Autodesk Inventor part; units mm, degrees
ref_plane "Plano de trabajo1" through (120, 0, 0) normal (1, 0, 0) x (0, 1, 0)
ref_plane "Plano de trabajo2" through (0, 0, -3) normal (0, 0, 1) x (1, 0, 0)
ref_plane "XZ Plane" through (0, 0, 0) normal (0, 1, 0) x (-1, 0, 0)
sketch "Boceto1" plane through (0, 0, 0) normal (0, 0, 1) x (1, 0, 0)
  circle A0 centre (80, 128) radius 1.85
  circle A1 centre (20, 128) radius 1.85
  circle A2 centre (80, 20) radius 1.85
  circle A3 centre (20, 20) radius 1.85
  line L0 (0, 0) -> (100, 0)
  line L1 (0, 148) -> (0, 0)
  line L2 (97, 3) -> (3, 3)
  line L3 (3, 3) -> (3, 145)
  line L4 (97, 145) -> (97, 3)
  line L5 (100, 0) -> (100, 148)
  line L6 (3, 145) -> (97, 145)
  line L7 (100, 148) -> (0, 148)
  circle A4 centre (20, 128) radius 4
  circle A5 centre (80, 128) radius 4
  circle A6 centre (20, 20) radius 4
  circle A7 centre (80, 20) radius 4
  dimension "d0" = 8
  dimension "d1" = 8
  dimension "d2" = 8
  dimension "d3" = 8
  dimension "d30" = 3.7
  dimension "d31" = 3.7
  dimension "d32" = 3.7
  dimension "d33" = 3.7
extrude "base1" add sketch "Boceto1" against normal blind 10 contours A0 | A1 | A2 | A3 | L1 L7 L5 L0 | L2 L3 L6 L4 | A4 | A5 | A6 | A7
extrude "base2" add sketch "Boceto1" along normal blind 3 contours A0 | A1 | A2 | A3 | L2 L3 L6 L4 | A4 | A5 | A6 | A7
extrude "Extrusión3" add sketch "Boceto1" along normal blind 48 contours L1 L7 L5 L0
sketch "Boceto2" plane through (100, 0, -10) normal (1, 0, 0) x (0, 0, -1)
  line L0 (-16, 10) -> (-86, 10)
  line L1 (-86, 10) -> (-86, 138)
  line L2 (-86, 138) -> (-16, 138)
  line L3 (-16, 138) -> (-16, 10)
  point P0 (-3, 0)
  point P1 (-51, 74)
  dimension "d10" = 70
  dimension "d11" = 128
extrude "Extrusión4" cut sketch "Boceto2" against normal blind 48
sketch "Boceto3" plane through (0, 0, 0) normal (1, 0, 0) x (0, 1, 0)
  point P0 (0, 0)
fillet "Empalme2" radius 2 8 edges at (3, 3, 25.5) (50, 3, 3) (3, 74, 3) (3, 145, 25.5) (50, 145, 3) (97, 145, 25.5) (97, 74, 3) (97, 3, 25.5)
fillet "Empalme2" radius 5 2 edges at (98.5, 138, 6) (98.5, 10, 6)
ref_plane "Plano de trabajo1" through (120, 0, 0) normal (1, 0, 0) x (0, 1, 0)
sketch "Boceto4" plane through (120, 0, 0) normal (1, 0, 0) x (0, 1, 0)
  arc A0 (0, 2.8284) -> (0.5858, 1.4142) centre (2, 2.8284) ccw
  line L0 (0, 48) -> (0, 2.8284)
  line L1 (5, -3) -> (0.5858, 1.4142)
  line L2 (5, -3) -> (143, -3)
  line L3 (143, -3) -> (147.4142, 1.4142)
  line L4 (148, 2.8284) -> (148, 48)
  arc A1 (147.4142, 1.4142) -> (148, 2.8284) centre (146, 2.8284) ccw
  line L5 (146, 48) -> (148, 48)
  line L6 (143, 48) -> (146, 48)
  line L7 (5, 48) -> (143, 48)
  line L8 (2, 48) -> (5, 48)
  line L9 (0, 48) -> (2, 48)
  arc A2 (10, 43) -> (5, 48) centre (5, 43) ccw
  line L10 (10, 18) -> (10, 43)
  arc A3 (10, 18) -> (15, 13) centre (15, 18) ccw
  line L11 (133, 13) -> (15, 13)
  arc A4 (133, 13) -> (138, 18) centre (133, 18) ccw
  line L12 (138, 43) -> (138, 18)
  arc A5 (143, 48) -> (138, 43) centre (143, 43) ccw
  point P0 (0, 0)
sketch "Boceto5" plane through (0, 0, 0) normal (0, 1, 0) x (-1, 0, 0)
  arc A0 (0, 46.5) -> (-1.5, 48) centre (-1.5, 46.5) ccw
  line L0 (-2, 48) -> (-1.5, 48)
  line L1 (-2, 48) -> (-98, 48)
  line L2 (0, 46.5) -> (0, 2.8284)
  arc A1 (-98.5, 48) -> (-100, 46.5) centre (-98.5, 46.5) ccw
  line L3 (-98.5, 48) -> (-98, 48)
  line L4 (-100, 2.8284) -> (-100, 46.5)
  arc A2 (-100, 2.8284) -> (-99.4142, 1.4142) centre (-98, 2.8284) ccw
  line L5 (-95, -3) -> (-99.4142, 1.4142)
  line L6 (-5, -3) -> (-95, -3)
  arc A3 (-0.5858, 1.4142) -> (0, 2.8284) centre (-2, 2.8284) ccw
  line L7 (-5, -3) -> (-0.5858, 1.4142)
  point P0 (0, 0)
extrude "Extrusión5" cut sketch "Boceto1" along normal blind 2 contours A0 | A1 | A2 | A3
ref_plane "Plano de trabajo2" through (0, 0, -3) normal (0, 0, 1) x (1, 0, 0)
sketch "Boceto6" plane through (0, 0, -3) normal (0, 0, 1) x (1, 0, 0)
  circle A0 centre (20, 128) radius 2
  circle A1 centre (20, 128) radius 2.3
  circle A2 centre (20, 20) radius 0.35
  circle A3 centre (20, 20) radius 2.3
  circle A4 centre (80, 20) radius 0.35
  circle A5 centre (80, 20) radius 2.3
  circle A6 centre (80, 128) radius 0.35
  circle A7 centre (80, 128) radius 2.3
  point P0 (0, 0)
  dimension "d29" = 4.6
  dimension "d34" = 4.6
  dimension "d35" = 4.6
  dimension "d36" = 4.6
extrude "Extrusión6" [suppressed]
properties part number "_3DPrint"
Source: CAD feature listing. Evaluate the final solid. Frame: model axes, mm. A direction names the side the tool comes from. Coordinates: 2 decimals unless noted, no trailing zeros. Loops run counter-clockwise (first coordinate to the right, second up) from the corner with the lowest first, then second, coordinate; pieces in that order, holes last. Notation, with made-up numbers: M 68.5,-33 L 79.5,-33 A31 cw 79.5,3 Z; hole C 60.5,-29 d3. An arc over 180 degrees is marked long. Answer in a Markdown table with one row per item.
Q1. Section D-D on x = 32.5. Return the cut outline in (y, z).
Answers below:
| item | result |
|---|---|
| outline | M 0,-10 L 148,-10 L 148,48 L 145,48 L 145,5 A2 cw 143,3 L 5,3 A2 cw 3,5 L 3,48 L 0,48 Z |
Q2. Section B-B on x = 80. Return the cut outline in (y, z).
Answers below:
| item | result |
|---|---|
| outline | M 0,-10 L 148,-10 L 148,48 L 145,48 L 145,5 A2 cw 143,3 L 5,3 A2 cw 3,5 L 3,48 L 0,48 Z; hole M 18.15,0 L 21.85,0 L 21.85,2 L 18.15,2 Z; hole M 126.15,0 L 129.85,0 L 129.85,2 L 126.15,2 Z |
Q3. Set-up query: faces 1 (the flat face through (49, 75, -10)), 2 (the cylindrical face through (98, 137, 8)), 3 (the flat face through (49, 145, 26)), 4 (the cylindrical face through (80.995, 126.44, 0.986)). Return all of +Z, -Z, +X, -X, +Y, -Y with unobstructed straight access to the full face (end or side cutting, diameter ignored); none if empty.
Answers below:
| item | result |
|---|---|
| face 1 | -Z, +X, -X, +Y, -Y |
| face 2 | +Z, +X |
| face 3 | +Z |
| face 4 | none |
Q4. Section C-C on y = 123. Return the cut outline in (x, z).
Answers below:
| item | result |
|---|---|
| outline | M 0,-10 L 100,-10 L 100,6 L 97,6 L 97,5 A2 cw 95,3 L 5,3 A2 cw 3,5 L 3,48 L 0,48 Z |
Q5. Draft query along Z for faces 5 (the flat face through (49, 75, 3)), 6 (the flat face through (20, 20, 0)), 7 (the flat face through (99, 138, 30)). Return one class per face: pulls with the +Z half, pulls with the -Z half, needs draft (parallel to the pull), parting line crosses it, or undercut.
Answers below:
| item | result |
|---|---|
| face 5 | pulls with the +Z half |
| face 6 | undercut |
| face 7 | needs draft |
Q6. Section A-A on y = 20. Return the cut outline in (x, z).
Answers below:
| item | result |
|---|---|
| outline | M 0,-10 L 100,-10 L 100,6 L 97,6 L 97,5 A2 cw 95,3 L 5,3 A2 cw 3,5 L 3,48 L 0,48 Z; hole M 18.15,0 L 21.85,0 L 21.85,2 L 18.15,2 Z; hole M 78.15,0 L 81.85,0 L 81.85,2 L 78.15,2 Z |
Q7. Ray query, probe 1 along Y at (x, z) = (20, 1.15); probe 2 along X at (y, z) = (128, 1.2); probe 3 along Y at (x, z) = (7, 31.5). Return the intervals inside material, ascending. Write a range as from..to.
Answers below:
| item | result |
|---|---|
| probe 1 | y = 0..18.15, 21.85..126.15, 129.85..148 |
| probe 2 | x = 0..18.15, 21.85..78.15, 81.85..100 |
| probe 3 | y = 0..3, 145..148 |
Q8. First-contact query: pin 1 (1.9 mm diameter, centred on x = 20.5, y = 20.5, fed in from +Z); pin 2 (3.5 mm diameter, centred on x = 99, y = 77, fed in from +Z). Flat tips, straight axial feed; report the tip coordinate or a pass-through.
Answers below:
| item | result |
|---|---|
| pin 1 | stops at z = 3 |
| pin 2 | stops at z = 6 |
